Read the model definition and answer for the solid it produces. Units are mm, in the model's axes. A direction names the side the tool comes from. Coordinates: 2 decimals unless noted, no trailing zeros. Write each loop counter-clockwise with the first axis right and the second up, starting at its lowest first coordinate (ties: lowest second). Pieces come first, ordered by that corner, then holes. Notation, with made-up numbers: (29, -14) -> (62, -14) arc R8 cw to (62, 1) -> close; hole circle Ø9 at (47.25, 10.5). An arc over 180 degrees is marked (long way). One line per item, written item: value. Start each with the question number.
1. Find section B-B, the plane y = -17.5. Write down the section's boundary in (x, z), and give its area (3 significant figures).
2. For a pull along Y with two mould halves and no side action, classify faces 1 (the flat face through (33, -21.5, 32)), 2 (the flat face through (0, 23, 42.3)), 3 (the cylindrical face through (-19.074, 0.496, -1.521)), 4 (the flat face through (0, 15, 0)) as pulls with the +Y half, pulls with the -Y half, needs draft (parallel to the pull), parting line crosses it, or undercut.
3. Find section D-D, the plane z = 55.3. Write down the section's boundary in (x, y).
4. For faces 5 (the flat face through (-24.5, -11, 32)), 6 (the flat face through (-9.5, 21, 54)), 7 (the flat face through (24.5, -11, 31)), determine the directions among +Z, -Z, +X, -X, +Y, -Y from which every point of the face is accessible in a straight line to the end or side of a thin tool.
5. Find section A-A, the plane z = 13.5. Write down the section's boundary in (x, y).
6. Find section C-C, the plane x = 33. Write down the section's boundary in (y, z), and give its area (3 significant figures).
7. Consider line 1 along Y through (x, z) = (0.5, 0.5); line 2 along Y through (x, z) = (30, 52.5); line 3 along X through (y, z) = (18, 40.5). Determine where each line is inside the solid, lowest interval first.
8. Given P1, Ø5, axis at x = 33, z = 55.3, coming from the +Y side; P2, Ø2, axis at y = 8, z = 8.5, coming from the -X side; P3, Ø2.5, axis at y = 20.5, z = 58.5, coming from the +X side, each flat-ended and moving along its own axis, determine where each tip first touches the part or whether it passes through.
```python
from build123d import *

# Parameters (mm, degrees)
ESQUISSE1_R             = 24.5
ESQUISSE1_R_2           = 21.5
BOSS_EXTRU_1_DEPTH      = 65.3
ESQUISSE2_R             = 21.5
ESQUISSE2_R_2           = 14.5
BOSS_EXTRU_2_DEPTH      = 3
ESQUISSE3_R             = 1.65
ENL_V_MAT_EXTRU_1_DEPTH = 3
ESQUISSE4_W             = 19
ESQUISSE4_H             = 5.738367338
ENL_V_MAT_EXTRU_2_DEPTH = 23
ESQUISSE5_W             = 68.3
ESQUISSE5_H             = 3
BOSS_EXTRU_3_DEPTH      = 17
ESQUISSE6_W             = 68.3
ESQUISSE6_H             = 3
BOSS_EXTRU_4_DEPTH      = 17
ESQUISSE7_R             = 2
ENL_V_MAT_EXTRU_3_DEPTH = 10
ESQUISSE9_R             = 2
ENL_V_MAT_EXTRU_4_DEPTH = 10


with BuildPart() as part:
    # Esquisse1 → Boss.-Extru.1 (new body)
    with BuildSketch(Plane.XY):
        Circle(ESQUISSE1_R)
        Circle(ESQUISSE1_R_2, mode=Mode.SUBTRACT)
        with BuildLine():
            Line((-24.5, 0), (-24.5, -24.5))
            Line((-24.5, -24.5), (-6e-09, -24.5))
            ThreePointArc((-6e-09, -24.5), (-17.324116141, -17.324116137), (-24.5, 0))
        make_face()
        with BuildLine():
            ThreePointArc((24.5, 0), (17.324116137, -17.324116141), (-6e-09, -24.5))
            Line((-6e-09, -24.5), (24.5, -24.5))
            Line((24.5, -24.5), (24.5, 0))
        make_face()
    extrude(amount=BOSS_EXTRU_1_DEPTH)

    # Esquisse2 → Boss.-Extru.2 (add)
    with BuildSketch(Plane(origin=(0, 0, 0), x_dir=(-1, 0, 0), z_dir=(0, 0, -1))):
        with BuildLine():
            ThreePointArc((24.5, 0), (0, 24.5), (-24.5, 0))
            ThreePointArc((-24.5, 0), (-17.324116141, -17.324116137), (-6e-09, -24.5))
            ThreePointArc((-6e-09, -24.5), (17.324116137, -17.324116141), (24.5, 0))
        make_face()
        with Locations(Location((0, 0, 0), (0, 0, 180))):
            Circle(ESQUISSE2_R, mode=Mode.SUBTRACT)
        with Locations(Location((0, 0, 0), (0, 0, 180))):
            Circle(ESQUISSE2_R)
        Circle(ESQUISSE2_R_2, mode=Mode.SUBTRACT)
        with BuildLine():
            ThreePointArc((-6e-09, -24.5), (-17.324116141, -17.324116137), (-24.5, 0))
            Line((-24.5, 0), (-24.5, -24.5))
            Line((-24.5, -24.5), (-6e-09, -24.5))
        make_face()
        with BuildLine():
            Line((24.5, -24.5), (24.5, 0))
            ThreePointArc((24.5, 0), (17.324116137, -17.324116141), (-6e-09, -24.5))
            Line((-6e-09, -24.5), (24.5, -24.5))
        make_face()
    extrude(amount=BOSS_EXTRU_2_DEPTH)

    # Esquisse3 → Enlèv. mat.-Extru.1 (cut)
    with BuildSketch(Plane(origin=(0, 0, -3), x_dir=(-1, 0, 0), z_dir=(0, 0, -1))):
        with Locations((-17.5, 0)):
            Circle(ESQUISSE3_R)
        with Locations((17.5, 0)):
            Circle(ESQUISSE3_R)
        with Locations((0, 17.5)):
            Circle(ESQUISSE3_R)
        with Locations((0, -17.5)):
            Circle(ESQUISSE3_R)
    extrude(amount=-ENL_V_MAT_EXTRU_1_DEPTH, mode=Mode.SUBTRACT)

    # Esquisse4 → Enlèv. mat.-Extru.2 (cut)
    with BuildSketch(Plane.XY.offset(65.3)):
        with Locations((0, 22.156485191)):
            Rectangle(ESQUISSE4_W, ESQUISSE4_H)
    extrude(amount=-ENL_V_MAT_EXTRU_2_DEPTH, mode=Mode.SUBTRACT)

    # Esquisse5 → Boss.-Extru.3 (add)
    with BuildSketch(Plane.ZY.offset(24.5)):
        with Locations((31.15, -23)):
            Rectangle(ESQUISSE5_W, ESQUISSE5_H)
    extrude(amount=BOSS_EXTRU_3_DEPTH)

    # Esquisse6 → Boss.-Extru.4 (add)
    with BuildSketch(Plane(origin=(24.5, 0, 0), x_dir=(0, 0, -1), z_dir=(1, 0, 0))):
        with Locations((-31.15, -23)):
            Rectangle(ESQUISSE6_W, ESQUISSE6_H)
    extrude(amount=BOSS_EXTRU_4_DEPTH)

    # Esquisse7 → Enlèv. mat.-Extru.3 (cut)
    with BuildSketch(Plane(origin=(0, -21.5, 0), x_dir=(1, 0, 0), z_dir=(0, 1, 0))):
        with Locations(Location((-33, -7, 0), (0, 0, 270))):
            Circle(ESQUISSE7_R)
        with Locations(Location((-33, -55.3, 0), (0, 0, 270))):
            Circle(ESQUISSE7_R)
    extrude(amount=-ENL_V_MAT_EXTRU_3_DEPTH, mode=Mode.SUBTRACT)

    # Esquisse9 → Enlèv. mat.-Extru.4 (cut)
    with BuildSketch(Plane(origin=(0, -21.5, 0), x_dir=(1, 0, 0), z_dir=(0, 1, 0))):
        with Locations(Location((33, -7, 0), (0, 0, 270))):
            Circle(ESQUISSE9_R)
        with Locations(Location((33, -55.3, 0), (0, 0, 270))):
            Circle(ESQUISSE9_R)
    extrude(amount=-ENL_V_MAT_EXTRU_4_DEPTH, mode=Mode.SUBTRACT)


solid = part.part
```
Answer block:
1. outline: (-24.5, -3) -> (-1.65, -3) -> (-1.65, 0) -> (-12.49, 0) -> (-12.49, 65.3) -> (-24.5, 65.3) -> close; (1.65, -3) -> (24.5, -3) -> (24.5, 65.3) -> (12.49, 65.3) -> (12.49, 0) -> (1.65, 0) -> close
1. area: 1,710 mm2
2. face 1: pulls with the +Y half
2. face 2: needs draft
2. face 3: undercut
2. face 4: undercut
3. outline: (-41.5, -24.5) -> (-35, -24.5) -> (-35, -21.5) -> (-41.5, -21.5) -> close; (-31, -24.5) -> (31, -24.5) -> (31, -21.5) -> (24.5, -21.5) -> (24.5, 0) arc R24.5 ccw to (9.5, 22.58) -> (9.5, 19.29) arc R21.5 cw (long way) to (-9.5, 19.29) -> (-9.5, 22.58) arc R24.5 ccw to (-24.5, 0) -> (-24.5, -21.5) -> (-31, -21.5) -> close; (35, -24.5) -> (41.5, -24.5) -> (41.5, -21.5) -> (35, -21.5) -> close
4. face 5: +Z, -Z, -X, +Y
4. face 6: +Z, +Y
4. face 7: +Z, -Z, +X, +Y
5. outline: (-41.5, -24.5) -> (41.5, -24.5) -> (41.5, -21.5) -> (24.5, -21.5) -> (24.5, 0) arc R24.5 ccw to (-24.5, 0) -> (-24.5, -21.5) -> (-41.5, -21.5) -> close; hole circle Ø43 at (0, 0)
6. outline: (-24.5, -3) -> (-21.5, -3) -> (-21.5, 5) -> (-24.5, 5) -> close; (-24.5, 9) -> (-21.5, 9) -> (-21.5, 53.3) -> (-24.5, 53.3) -> close; (-24.5, 57.3) -> (-21.5, 57.3) -> (-21.5, 65.3) -> (-24.5, 65.3) -> close
6. area: 181 mm2
7. line 1: y = -24.5 to -21.49, 21.49 to 24.49
7. line 2: y = -24.5 to -21.5
7. line 3: x = -16.62 to -11.76, 11.76 to 16.62
8. P1: stops at y = -21.5
8. P2: stops at x = -23.48
8. P3: stops at x = 15.16
